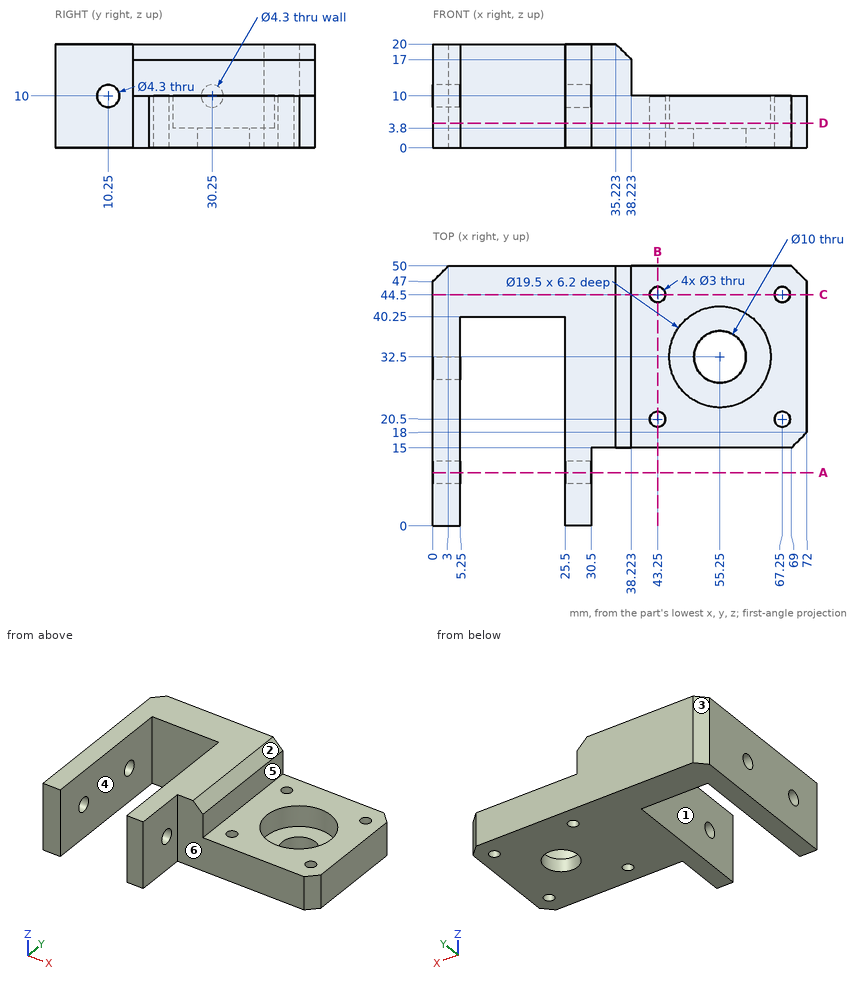
Answer from the drawing. Dimensions are ordinates in mm from the lowest x, y and z of the part. A direction names the side the tool comes from. Round coordinates to 2 decimals unless told otherwise and drop trailing zeros. Write each loop counter-clockwise with the first axis right and the second up, starting at its lowest first coordinate (ties: lowest second). Pieces come first, ordered by that corner, then holes. Notation, with made-up numbers: M 36.5,-2 L 87.5,-2 A12 ccw 87.5,5 Z; hole C -12,20.25 d8. An arc over 180 degrees is marked long. Write each question's results on one line, items separated by ' | '. Start each with the question number.
Item 1: Find section A-A on y = 10.25. Write down the section's boundary in (x, z).
Item 2: Which of the six approach directions +Z, -Z, +X, -X, +Y, -Y give full straight-line access (tool end or side, diameter ignored) to the marked faces 4, 5 and 6?
Item 3: The mould has two halves that part along X. Classify the marked faces 1, 2 and 3: +X half, -X half, draft (parallel to the pull), parting line (faces both ways), or undercut.
Item 4: Find section B-B on x = 43.25. Write down the section's boundary in (y, z).
Item 5: Find section C-C on y = 44.5. Write down the section's boundary in (x, z).
Item 6: Straight lines are drawn through the part: probe 1 along Y at (x, z) = (43.25, 3.75); probe 2 along X at (y, z) = (20.5, 6.25); probe 3 along X at (y, z) = (44.5, 4.25). For each, find the intervals that lie inside material, in ascending order.
Item 7: Find section D-D on z = 4.75. Write down the section's boundary in (x, y), and give its area (3 significant figures).
Item 8: Given pin 1 Ø15.5 at (x, y) = (51, 36) entering from +Z; pin 2 Ø4.5 at (y, z) = (4.5, 11) entering from +X; pin 3 Ø6 at (y, z) = (16, 11) entering from +X; pin 4 Ø5 at (x, z) = (19, 5.5) entering from -Y, each flat-ended and moving along its own axis, determine where each tip first touches the part or whether it passes through.
Answer block:
1) outline: M 0,0 L 5.25,0 L 5.25,7.85 L 0,7.85 Z; M 0,12.15 L 5.25,12.15 L 5.25,20 L 0,20 Z; M 25.5,0 L 30.5,0 L 30.5,7.85 L 25.5,7.85 Z; M 25.5,12.15 L 30.5,12.15 L 30.5,20 L 25.5,20 Z
2) face 4: +Z, -Z, -Y | face 5: +Z, +X, +Y, -Y | face 6: +Z, -Z, +X, -Y
3) face 1: undercut | face 2: +X half | face 3: -X half
4) outline: M 15,0 L 19,0 L 19,10 L 15,10 Z; M 22,0 L 43,0 L 43,10 L 22,10 Z; M 46,0 L 50,0 L 50,10 L 46,10 Z
5) outline: M 0,0 L 41.75,0 L 41.75,10 L 38.22,10 L 38.22,17 L 35.22,20 L 0,20 Z; M 44.75,0 L 65.75,0 L 65.75,10 L 44.75,10 Z; M 68.75,0 L 72,0 L 72,10 L 68.75,10 Z
6) probe 1: y = 15 to 19, 22 to 43, 46 to 50 | probe 2: x = 0 to 5.25, 25.5 to 41.75, 44.75 to 65.75, 68.75 to 72 | probe 3: x = 0 to 41.75, 44.75 to 65.75, 68.75 to 72
7) outline: M 0,0 L 5.25,0 L 5.25,40.25 L 25.5,40.25 L 25.5,0 L 30.5,0 L 30.5,15 L 69,15 L 72,18 L 72,47 L 69,50 L 3,50 L 0,47 Z; hole C 43.25,20.5 d3; hole C 43.25,44.5 d3; hole C 55.25,32.5 d19.5; hole C 67.25,20.5 d3; hole C 67.25,44.5 d3 | area: 1,820 mm²
8) pin 1: stops at z = 10 | pin 2: stops at x = 30.5 | pin 3: stops at x = 72 | pin 4: stops at y = 40.25
